Part print with two shaded views. Sizes in mm from the minimum x, y, z corner. A direction names the side the tool comes from. Round coordinates to 2 decimals unless told otherwise and drop trailing zeros. Loops run counter-clockwise (first coordinate to the right, second up) from the corner with the lowest first, then second, coordinate; pieces in that order, holes last.
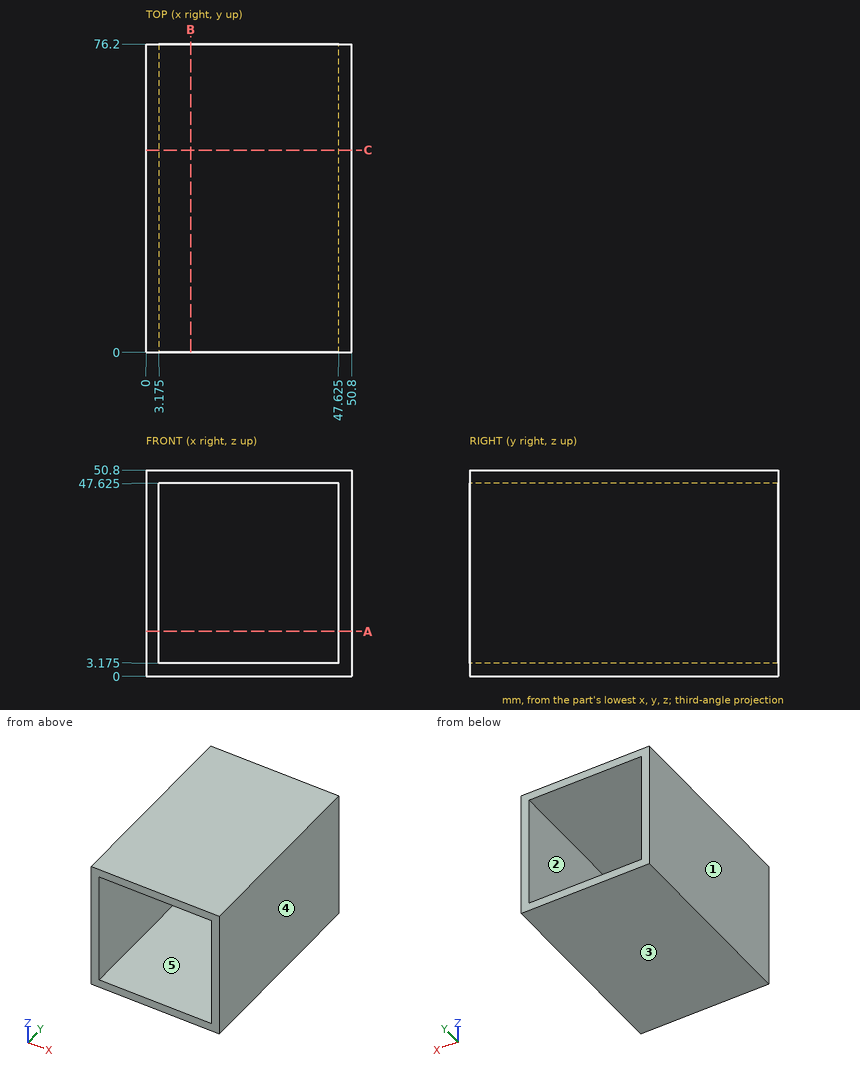
Item 1: Cut at C-C (y = 50). List the corners of the cut face in (x, z) (3 decimals), plus the area to 3 significant figures.
Verdict:
outline: (0, 0) - (50.8, 0) - (50.8, 50.8) - (0, 50.8) - close; hole (3.175, 3.175) - (47.625, 3.175) - (47.625, 47.625) - (3.175, 47.625) - close
area: 605 mm2
Item 2: Cut at B-B (x = 11). List the corners of the cut face in (y, z) (3 decimals), plus the area to 3 significant figures.
Verdict:
outline: (0, 0) - (76.2, 0) - (76.2, 3.175) - (0, 3.175) - close; (0, 47.625) - (76.2, 47.625) - (76.2, 50.8) - (0, 50.8) - close
area: 484 mm2
Item 3: 3-axis set-ups, long thin cutter, end or side, ignore diameter. For the marked faces 4 and 5: which of +Z, -Z, +X, -X, +Y, -Y reach the whole face in a straight line?
Verdict:
face 4: +Z, -Z, +X, +Y, -Y
face 5: +Y, -Y
Item 4: Mould opens along X. For the marked faces 1, 2 and 3 say: released by +X, released by -X, zero draft, split by the parting line, or undercut.
Verdict:
face 1: released by -X
face 2: undercut
face 3: zero draft
Item 5: Cut at A-A (z = 11). List the corners of the cut face in (x, y) (3 decimals).
Verdict:
outline: (0, 0) - (3.175, 0) - (3.175, 76.2) - (0, 76.2) - close; (47.625, 0) - (50.8, 0) - (50.8, 76.2) - (47.625, 76.2) - close
Item 6: Wall check: L1, parallel to Z at x = 21.5, y = 37.5 (3 decimals). Give the ranges that are in metal, low to high.
Verdict:
L1: z = 0 to 3.175, 47.625 to 50.8
